Autodesk Fusion 360 part; units mm, degrees
sketch "Sketch1" plane through (0, 0, 0) normal (0, 0, 1) x (1, 0, 0)
  line L0 (22.5, 22.5) -> (-22.5, 22.5)
  line L1 (-20, 20) -> (-20, 10)
  line L2 (22.5, -22.5) -> (22.5, 22.5)
  line L3 (20, -20) -> (10, -20)
  line L4 (-22.5, 22.5) -> (-22.5, -22.5)
  line L5 (-20, -20) -> (10, -20)
  line L6 (-20, 20) -> (-22.5, 22.5)
  line L7 (20, -20) -> (20, 20)
  line L8 (20, -20) -> (22.5, -22.5)
  line L9 (-20, 10) -> (-20, -20)
  line L10 (20, 20) -> (-20, 20)
  line L11 (-22.5, -22.5) -> (22.5, -22.5)
  line L12 (-18.5858, -20) -> (0, -1.4142)
  line L13 (1.4142, 0) -> (20, 18.5858)
  line L14 (18.5858, -20) -> (0, -1.4142)
  line L15 (-1.4142, 0) -> (-20, 18.5858)
  line L16 (-20, -18.5858) -> (-1.4142, 0)
  line L17 (0, 1.4142) -> (18.5858, 20)
  line L18 (20, -18.5858) -> (1.4142, 0)
  line L19 (0, 1.4142) -> (-18.5858, 20)
  line L20 (-18.5858, -20) -> (0, -1.4142)
  line L21 (1.4142, 0) -> (20, 18.5858)
  line L22 (-20, -18.5858) -> (-1.4142, 0)
  line L23 (0, 1.4142) -> (18.5858, 20)
  line L24 (20, -13.636) -> (6.364, 0)
  line L25 (0, 6.364) -> (-13.636, 20)
  line L26 (-20, -13.636) -> (-6.364, 0)
  line L27 (0, 6.364) -> (13.636, 20)
  line L28 (13.636, -20) -> (0, -6.364)
  line L29 (-6.364, 0) -> (-20, 13.636)
  line L30 (-20, -13.636) -> (-6.364, 0)
  line L31 (0, 6.364) -> (13.636, 20)
  line L32 (-13.636, -20) -> (0, -6.364)
  line L33 (6.364, 0) -> (20, 13.636)
  line L34 (6.364, 0) -> (20, 13.636)
  line L35 (-13.636, -20) -> (0, -6.364)
  line L36 (-20, -20) -> (-22.5, -22.5)
  line L37 (20, 20) -> (22.5, 22.5)
  dimension "d3" = 45
  dimension "d4" = 45
extrude "Extrude1" add sketch "Sketch1" along normal blind 3 contours L0 L6 L10 L37 | L2 L7 L8 L37 | L1 L4 L6 L9 L36 | L3 L5 L8 L11 L36 | L7 L13 L18 L21 L24 L33 L34 | L10 L17 L19 L23 L25 L27 L31 | L1 L9 L15 L16 L22 L26 L29 L30 | L3 L5 L12 L14 L20 L28 L32 L35
fillet "Fillet1" radius 2 12 edges at (-20, 13.636, 1.5) (-20, -13.636, 1.5) (-6.364, 0, 1.5) (0, -6.364, 1.5) (20, 13.636, 1.5) (-13.636, -20, 1.5) (6.364, 0, 1.5) (0, 6.364, 1.5) (13.636, -20, 1.5) (20, -13.636, 1.5) (13.636, 20, 1.5) (-13.636, 20, 1.5)
extrude "Extrude2" add sketch "Sketch1" against normal blind 15 contours L3 L5 L8 L11 L36
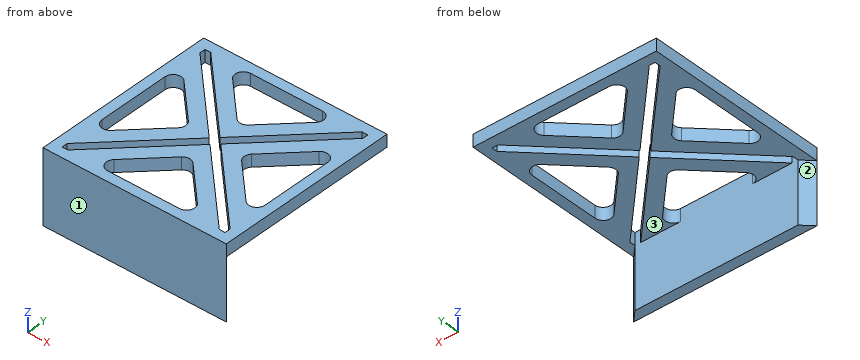
For this review, take the finished solid that the model builds, in its own axes (mm). Face numbers are marked on the shaded views. A direction names the side the tool comes from. Round coordinates to 2 decimals unless told otherwise and drop trailing zeros. Loops run counter-clockwise (first coordinate to the right, second up) from the corner with the lowest first, then second, coordinate; pieces in that order, holes last. Notation, with made-up numbers: (8.5, 46.5) - (62.5, 46.5) arc R21 ccw to (62.5, 55.5) - close; hole circle Ø8 at (69, 68). An arc over 180 degrees is marked (long way). Answer as CSV lines item,"result".
(1) Consider section C-C on x = 15.5. Give the boundary of the cut face in (y, z).
Checked values:
outline,"(-22.5, -15) - (-20, -15) - (-20, 0) - (-16.91, 0) - (-16.91, 3) - (-22.5, 3) - close; (-14.09, 0) - (-9.14, 0) - (-9.14, 3) - (-14.09, 3) - close; (9.14, 0) - (14.09, 0) - (14.09, 3) - (9.14, 3) - close; (16.91, 0) - (22.5, 0) - (22.5, 3) - (16.91, 3) - close"
(2) Wall thickness on line 1 (X direction, y = 4.5, z = 2); line 2 (Y direction, x = -11.5, z = 1.75); line 3 (Y direction, x = -6, z = 1): over which ranges is each line inside the solid? List them lowest first.
Checked values:
line 1,"x = -22.5 to -20, -10.86 to -5.91, -3.09 to 3.09, 5.91 to 10.86, 20 to 22.5"
line 2,"y = -22.5 to -12.91, -10.09 to -5.14, 5.14 to 10.09, 12.91 to 22.5"
line 3,"y = -22.5 to -20, -12.36 to -7.41, -4.59 to 4.59, 7.41 to 12.36, 20 to 22.5"
(3) Consider section B-B on x = -6. Give the boundary of the cut face in (y, z).
Checked values:
outline,"(-22.5, -15) - (-20, -15) - (-20, 3) - (-22.5, 3) - close; (-12.36, 0) - (-7.41, 0) - (-7.41, 3) - (-12.36, 3) - close; (-4.59, 0) - (4.59, 0) - (4.59, 3) - (-4.59, 3) - close; (7.41, 0) - (12.36, 0) - (12.36, 3) - (7.41, 3) - close; (20, 0) - (22.5, 0) - (22.5, 3) - (20, 3) - close"
(4) Insertion check: P1, Ø9.5, axis at x = -5.5, y = -6.5, coming from the -Z side; P2, Ø5.5, axis at x = 4.5, z = -8.5, coming from the +Y side; P3, Ø1, axis at x = 0.5, y = -18, coming from the -Z side. Each pin has a flat end and moves straight along its axis. Give the tip position at first contact, or say it passes through.
Checked values:
P1,"stops at z = 0"
P2,"stops at y = -20"
P3,"passes through"
(5) Tool access review of the marked faces 1, 2 and 3: name each direction out of +Z, -Z, +X, -X, +Y, -Y from which nothing blocks a thin tool from reaching the whole face with its end or side.
Checked values:
face 1,"+Z, -Z, +X, -X, -Y"
face 2,"-Z, -X, +Y"
face 3,"-Z, +X, -X, +Y"
(6) Consider section A-A on y = -5. Give the boundary of the cut face in (x, z), then the cut area to 3 significant figures.
Checked values:
outline,"(-22.5, 0) - (-20, 0) - (-20, 3) - (-22.5, 3) - close; (-11.36, 0) - (-6.41, 0) - (-6.41, 3) - (-11.36, 3) - close; (-3.59, 0) - (3.59, 0) - (3.59, 3) - (-3.59, 3) - close; (6.41, 0) - (11.36, 0) - (11.36, 3) - (6.41, 3) - close; (20, 0) - (22.5, 0) - (22.5, 3) - (20, 3) - close"
area,"66.2 mm2"
(7) Consider section D-D on y = -13. Give the boundary of the cut face in (x, z).
Checked values:
outline,"(-22.5, 0) - (-14.41, 0) - (-14.41, 3) - (-22.5, 3) - close; (-11.59, 0) - (-6.64, 0) - (-6.64, 3) - (-11.59, 3) - close; (6.64, 0) - (11.59, 0) - (11.59, 3) - (6.64, 3) - close; (14.41, 0) - (22.5, 0) - (22.5, 3) - (14.41, 3) - close"
